Geometry: final body of the model. Coordinates: model frame, mm. A direction names the side the tool comes from. Give positions to 0.01 mm unless a question says otherwise; leave off trailing zeros. Write each loop counter-clockwise with the first axis right and the second up, starting at its lowest first coordinate (ties: lowest second). Pieces come first, ordered by that corner, then holes.
Q1. Section B-B (x = 0). Return the cut outline in (y, z), plus the area to 3 significant figures.
Q2. Reachability of faces 1 (the flat face through (-0.5, -2, -10)), 2 (the flat face through (-2, 0.6, 4)), 3 (the flat face through (0, -2.6, 2.65)), 4 (the flat face through (0.5, 2, 10)) from +Z, -Z, +X, -X, +Y, -Y: full face, straight path, thin tool, end or side. Return the list, or none.
Q3. Line query: line 1 (Z direction, x = -2.25, y = -0.7); line 2 (Y direction, x = 0, z = -1.5); line 3 (Y direction, x = 1, z = 10.75). Output: solid intervals per line, ascending.
Q4. Section D-D (y = 1.2). Return the cut outline in (x, z).
Q5. Mould query, pull axis Z, two halves, no side actions, for faces 5 (the cylindrical face through (0.06, 2.95, 3.82)), 6 (the flat face through (-2, 0, 11.95)), 7 (the flat face through (0, 2.6, 4.95)), 8 (the flat face through (0.2, -2.5, 4.95)). Classes: +Z half, -Z half, draft (parallel to the pull), parting line (faces both ways), or undercut.
Q6. Section A-A (y = 0). State how many separate pieces and enclosed holes the cut face has, plus the area to 3 significant figures.
Q7. Section C-C (z = 6.25). Return the cut outline in (x, y).
Q8. Pin query (flat end, axial travel): pin 1 Ø1 at (y, z) = (-2, -11) entering from -X; pin 2 Ø0.7 at (x, z) = (-2.5, 2.5) entering from +Y; pin 3 Ø0.5 at (y, z) = (2, -10) entering from +X. Return the tip coordinate at first contact, or that it passes through.
from build123d import *

# Parameters (mm, degrees)
F0_R      = 2.95
F1_DEPTH  = 11.95
F2_R      = 2.95
F2_R_2    = 2.3
F3_DEPTH  = 7
F4_R      = 2.95
F4_R_2    = 2.3
F5_DEPTH  = 14.6
F6_R      = 1.6
F7_DEPTH  = 23.901
F9_DEPTH  = 12.5
F10_W     = 0.2
F10_H     = 0.2
F12_DEPTH = 12.5
F13_DEPTH = 12.5
F15_DEPTH = 12.5


# Not quite as in the source:
# - a pattern or mirror of a feature is missing from the dataset's text; its kind, count and spacing are read off the source's solid


with BuildPart() as f1:
    # F0 (on Top) → F1 (new body, symmetric)
    with BuildSketch(Plane.XY):
        Circle(F0_R)
    extrude(amount=F1_DEPTH, both=True)

    # F2 (on face) → F3 (cut)
    with BuildSketch(Plane.XY.offset(11.95)):
        Circle(F2_R)
        Circle(F2_R_2, mode=Mode.SUBTRACT)
    extrude(amount=-F3_DEPTH, mode=Mode.SUBTRACT)

    # F4 (on face) → F5 (cut)
    with BuildSketch(Plane(origin=(0, 0, -11.95), x_dir=(1, 0, 0), z_dir=(0, 0, -1))):
        Circle(F4_R)
        Circle(F4_R_2, mode=Mode.SUBTRACT)
    extrude(amount=-F5_DEPTH, mode=Mode.SUBTRACT)

    # F6 (on face) → F7 (cut, through all)
    with BuildSketch(Plane.XY.offset(11.95)):
        Circle(F6_R)
    extrude(amount=-F7_DEPTH, mode=Mode.SUBTRACT)

    # F8 (on Front) → F9 (cut, symmetric)
    with BuildSketch(Plane.XZ):
        with BuildLine():
            ThreePointArc((0.5, 8.8), (0, 9.3), (-0.5, 8.8))
            Line((-0.5, 8.8), (0.5, 8.8))
        make_face()
        with BuildLine():
            Line((-0.5, 11.95), (-0.5, 8.8))
            ThreePointArc((-0.5, 8.8), (0, 9.3), (0.5, 8.8))
            Line((0.5, 8.8), (0.5, 11.95))
            Line((0.5, 11.95), (-0.5, 11.95))
        make_face()
        with BuildLine():
            Line((0.5, 8.8), (-0.5, 8.8))
            ThreePointArc((-0.5, 8.8), (0, 8.3), (0.5, 8.8))
        make_face()
        with BuildLine():
            Line((-0.5, -8.8), (-0.5, -11.95))
            Line((-0.5, -11.95), (0.5, -11.95))
            Line((0.5, -11.95), (0.5, -8.8))
            ThreePointArc((0.5, -8.8), (0, -9.3), (-0.5, -8.8))
        make_face()
        with BuildLine():
            ThreePointArc((0.5, -8.8), (0, -8.3), (-0.5, -8.8))
            Line((-0.5, -8.8), (0.5, -8.8))
        make_face()
        with BuildLine():
            Line((0.5, -8.8), (-0.5, -8.8))
            ThreePointArc((-0.5, -8.8), (0, -9.3), (0.5, -8.8))
        make_face()
    extrude(amount=F9_DEPTH, both=True, mode=Mode.SUBTRACT)

    # F10 (on Front) → F11 (revolve)
    with BuildSketch(Plane.XZ):
        with Locations((2.4, 11.85)):
            Rectangle(F10_W, F10_H)
    f11 = revolve(axis=Axis((0, 0, 11.95), (0, 0, 1)))

    # F11_copies: F11 across plane
    add(f11.mirror(Plane(origin=(0, 0, 0), x_dir=(-1, 0, 0), z_dir=(0, 0, -1))))

    # F8 (on Front) → F12 (cut, symmetric)
    with BuildSketch(Plane.XZ):
        with BuildLine():
            ThreePointArc((0.5, 8.8), (0, 9.3), (-0.5, 8.8))
            Line((-0.5, 8.8), (0.5, 8.8))
        make_face()
        with BuildLine():
            Line((-0.5, 11.95), (-0.5, 8.8))
            ThreePointArc((-0.5, 8.8), (0, 9.3), (0.5, 8.8))
            Line((0.5, 8.8), (0.5, 11.95))
            Line((0.5, 11.95), (-0.5, 11.95))
        make_face()
        with BuildLine():
            Line((0.5, 8.8), (-0.5, 8.8))
            ThreePointArc((-0.5, 8.8), (0, 8.3), (0.5, 8.8))
        make_face()
        with BuildLine():
            Line((-0.5, -8.8), (-0.5, -11.95))
            Line((-0.5, -11.95), (0.5, -11.95))
            Line((0.5, -11.95), (0.5, -8.8))
            ThreePointArc((0.5, -8.8), (0, -9.3), (-0.5, -8.8))
        make_face()
        with BuildLine():
            ThreePointArc((0.5, -8.8), (0, -8.3), (-0.5, -8.8))
            Line((-0.5, -8.8), (0.5, -8.8))
        make_face()
        with BuildLine():
            Line((0.5, -8.8), (-0.5, -8.8))
            ThreePointArc((-0.5, -8.8), (0, -9.3), (0.5, -8.8))
        make_face()
    extrude(amount=F12_DEPTH, both=True, mode=Mode.SUBTRACT)

    # F8 (on Front) → F13 (cut, symmetric)
    with BuildSketch(Plane.XZ):
        with BuildLine():
            ThreePointArc((0.5, 8.8), (0, 9.3), (-0.5, 8.8))
            Line((-0.5, 8.8), (0.5, 8.8))
        make_face()
        with BuildLine():
            Line((-0.5, 11.95), (-0.5, 8.8))
            ThreePointArc((-0.5, 8.8), (0, 9.3), (0.5, 8.8))
            Line((0.5, 8.8), (0.5, 11.95))
            Line((0.5, 11.95), (-0.5, 11.95))
        make_face()
        with BuildLine():
            Line((0.5, 8.8), (-0.5, 8.8))
            ThreePointArc((-0.5, 8.8), (0, 8.3), (0.5, 8.8))
        make_face()
        with BuildLine():
            Line((-0.5, -8.8), (-0.5, -11.95))
            Line((-0.5, -11.95), (0.5, -11.95))
            Line((0.5, -11.95), (0.5, -8.8))
            ThreePointArc((0.5, -8.8), (0, -9.3), (-0.5, -8.8))
        make_face()
        with BuildLine():
            ThreePointArc((0.5, -8.8), (0, -8.3), (-0.5, -8.8))
            Line((-0.5, -8.8), (0.5, -8.8))
        make_face()
        with BuildLine():
            Line((0.5, -8.8), (-0.5, -8.8))
            ThreePointArc((-0.5, -8.8), (0, -9.3), (0.5, -8.8))
        make_face()
    extrude(amount=F13_DEPTH, both=True, mode=Mode.SUBTRACT)

    # F14 (on Right) → F15 (cut, symmetric)
    with BuildSketch(Plane.YZ):
        with BuildLine():
            ThreePointArc((-0.6, 0.6), (0, 0), (0.6, 0.6))
            Line((0.6, 0.6), (-0.6, 0.6))
        make_face()
        with BuildLine():
            ThreePointArc((-0.6, 0.6), (0, 1.2), (0.6, 0.6))
            Line((0.6, 0.6), (0.6, 6.5))
            ThreePointArc((0.6, 6.5), (0, 5.9), (-0.6, 6.5))
            Line((-0.6, 6.5), (-0.6, 0.6))
        make_face()
        with BuildLine():
            Line((-0.6, 0.6), (0.6, 0.6))
            ThreePointArc((0.6, 0.6), (0, 1.2), (-0.6, 0.6))
        make_face()
        with BuildLine():
            ThreePointArc((-0.6, 6.5), (0, 5.9), (0.6, 6.5))
            Line((0.6, 6.5), (-0.6, 6.5))
        make_face()
        with BuildLine():
            Line((-0.6, 6.5), (0.6, 6.5))
            ThreePointArc((0.6, 6.5), (0, 7.1), (-0.6, 6.5))
        make_face()
        with BuildLine():
            ThreePointArc((-0.6, -7.1), (0, -7.7), (0.6, -7.1))
            Line((0.6, -7.1), (-0.6, -7.1))
        make_face()
        with BuildLine():
            ThreePointArc((-0.6, -7.1), (0, -6.5), (0.6, -7.1))
            Line((0.6, -7.1), (0.6, -1.2))
            ThreePointArc((0.6, -1.2), (0, -1.8), (-0.6, -1.2))
            Line((-0.6, -1.2), (-0.6, -7.1))
        make_face()
        with BuildLine():
            Line((-0.6, -7.1), (0.6, -7.1))
            ThreePointArc((0.6, -7.1), (0, -6.5), (-0.6, -7.1))
        make_face()
        with BuildLine():
            ThreePointArc((-0.6, -1.2), (0, -1.8), (0.6, -1.2))
            Line((0.6, -1.2), (-0.6, -1.2))
        make_face()
        with BuildLine():
            Line((-0.6, -1.2), (0.6, -1.2))
            ThreePointArc((0.6, -1.2), (0, -0.6), (-0.6, -1.2))
        make_face()
    extrude(amount=F15_DEPTH, both=True, mode=Mode.SUBTRACT)


solid = f1.part
Computed:
1. outline: (-2.95, 2.65) - (-2.3, 2.65) - (-2.3, -8.3) - (-1.6, -8.3) - (-1.6, 8.3) - (-2.3, 8.3) - (-2.3, 4.95) - (-2.95, 4.95) - close; (1.6, -8.3) - (2.3, -8.3) - (2.3, 2.65) - (2.95, 2.65) - (2.95, 4.95) - (2.3, 4.95) - (2.3, 8.3) - (1.6, 8.3) - close
1. area: 26.2 mm2
2. face 1: -Z, +Y, -Y
2. face 2: +X, -X
2. face 3: -Y
2. face 4: +Z, +Y, -Y
3. line 1: z = -11.95 to -11.75, 2.65 to 4.95, 11.75 to 11.95
3. line 2: y = -2.3 to -1.6, 1.6 to 2.3
3. line 3: y = -2.07 to -1.25, 1.25 to 2.07
4. outline: (-2.69, 2.65) - (-1.96, 2.65) - (-1.96, -11.75) - (-2.19, -11.75) - (-2.19, -11.95) - (-1.06, -11.95) - (-1.06, 11.95) - (-2.19, 11.95) - (-2.19, 11.75) - (-1.96, 11.75) - (-1.96, 4.95) - (-2.69, 4.95) - close; (1.06, -11.95) - (2.19, -11.95) - (2.19, -11.75) - (1.96, -11.75) - (1.96, 2.65) - (2.69, 2.65) - (2.69, 4.95) - (1.96, 4.95) - (1.96, 11.75) - (2.19, 11.75) - (2.19, 11.95) - (1.06, 11.95) - close
5. face 5: draft
5. face 6: +Z half
5. face 7: undercut
5. face 8: undercut
6. separate pieces: 6
6. enclosed holes: 0
6. area: 13.7 mm2
7. outline: (-2.22, -0.6) arc R2.3 ccw to (2.22, -0.6) - (1.48, -0.6) arc R1.6 cw to (-1.48, -0.6) - close; (-2.22, 0.6) - (-1.48, 0.6) arc R1.6 cw to (1.48, 0.6) - (2.22, 0.6) arc R2.3 ccw to start
8. pin 1: stops at x = -1.74
8. pin 2: stops at y = 1.98
8. pin 3: stops at x = 1.49
